The drawing under review shows one solid part. Ordinate dimensions are in mm from its lowest x, y, z. Coordinates: 2 decimals unless noted, no trailing zeros. Write each loop counter-clockwise with the first axis right and the second up, starting at its lowest first coordinate (ties: lowest second). Pieces come first, ordered by that corner, then holes. Notation, with made-up numbers: (68, 74.5) -> (72, 74.5) arc R23 ccw to (72, 105.5) -> close; hole circle Ø11 at (78, 11.25). An arc over 180 degrees is marked (long way). One line per item, written item: value. Start each with the question number.
1) Add section C-C (y = 36.5). State the section outline as (x, z) points.
2) Add section A-A (x = 86). State the section outline as (y, z) points.
3) Add section B-B (z = 1). State the section outline as (x, y) points, and give its area (3 significant figures).
4) For probe 1 along Y at (x, z) = (90.9, 0.4); probe 2 along Y at (x, z) = (90, 1); probe 3 along X at (y, z) = (33.5, 0.8), list the stretches that pass through material, from the lowest coordinate up. Write a range as from..to.
5) For pin 1 Ø0.9 at (x, y) = (90.9, 10.22) entering from +Z; pin 2 Ø0.5 at (y, z) = (30.5, 1) entering from +X, all flat-tipped, find the tip position at first contact; note any pin that passes through.
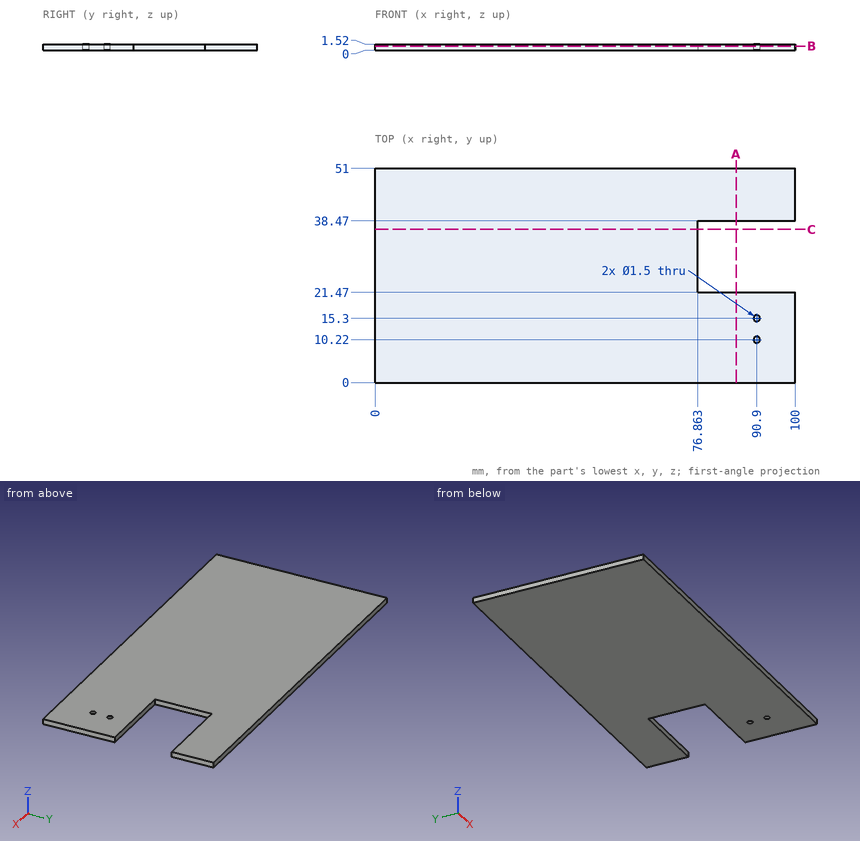
Numbers:
1. outline: (0, 0) -> (76.86, 0) -> (76.86, 1.52) -> (0, 1.52) -> close
2. outline: (0, 0) -> (21.47, 0) -> (21.47, 1.52) -> (0, 1.52) -> close; (38.47, 0) -> (51, 0) -> (51, 1.52) -> (38.47, 1.52) -> close
3. outline: (0, 0) -> (100, 0) -> (100, 21.47) -> (76.86, 21.47) -> (76.86, 38.47) -> (100, 38.47) -> (100, 51) -> (0, 51) -> close; hole circle Ø1.5 at (90.9, 10.22); hole circle Ø1.5 at (90.9, 15.3)
3. area: 4,700 mm²
4. probe 1: 0..9.47, 10.97..14.55, 16.05..21.47, 38.47..51
4. probe 2: 0..21.47, 38.47..51
4. probe 3: 0..76.86
5. pin 1: through
5. pin 2: x = 76.86
